```python
from build123d import *

# Parameters (mm, degrees)
SKETCH1_W           = 150
SKETCH1_H           = 150
BOSS_EXTRUDE1_DEPTH = 19
SKETCH2_R           = 28
CUT_EXTRUDE1_DEPTH  = 3
SKETCH3_R           = 2.5
CUT_EXTRUDE2_DEPTH  = 5
CIRPATTERN1_COUNT   = 4


with BuildPart() as part:
    # Sketch1 → Boss-Extrude1 (new body)
    with BuildSketch(Plane(origin=(0, 0, 0), x_dir=(1, 0, 0), z_dir=(0, 1, 0))):
        with Locations((75, 75)):
            Rectangle(SKETCH1_W, SKETCH1_H)
    extrude(amount=BOSS_EXTRUDE1_DEPTH)

    # Sketch2 → Cut-Extrude1 (cut)
    with BuildSketch(Plane(origin=(0, 19, 0), x_dir=(1, 0, 0), z_dir=(0, 1, 0))):
        with Locations((75, 75)):
            Circle(SKETCH2_R)
    extrude(amount=-CUT_EXTRUDE1_DEPTH, mode=Mode.SUBTRACT)

    # Sketch3 → Cut-Extrude2 (cut)
    with BuildSketch(Plane(origin=(0, 19, 0), x_dir=(1, 0, 0), z_dir=(0, 1, 0))):
        with Locations((100, 5)):
            Circle(SKETCH3_R)
        with Locations((50, 5)):
            Circle(SKETCH3_R)
    cut_extrude2 = extrude(amount=-CUT_EXTRUDE2_DEPTH, mode=Mode.SUBTRACT)

    # CirPattern1: Cut-Extrude2 ×4 about axis
    cirpattern1_axis = Axis((75, 0, -75), (0, 1, 0))
    for i in range(1, CIRPATTERN1_COUNT):
        add(cut_extrude2.rotate(cirpattern1_axis, i * 360 / CIRPATTERN1_COUNT), mode=Mode.SUBTRACT)


solid = part.part
```
Work out the finished part from the listing and answer in its coordinate system (mm). A direction names the side the tool comes from. Coordinates: 2 decimals unless noted, no trailing zeros. Write each loop counter-clockwise with the first axis right and the second up, starting at its lowest first coordinate (ties: lowest second). Pieces come first, ordered by that corner, then holes.
Q1. A cutting plane is placed at C-C, the plane z = -82.5. Give the vertices of the cut face in (x, y), then the cut area to 3 significant figures.
Q2. Find the intervals of material crossed by line 1 (Z direction, x = 145, y = 16.05); line 2 (X direction, y = 15.15, z = -5); line 3 (Z direction, x = 50, y = 15.65), in increasing order.
Q3. Each of these flat-tipped pins is pushed along its axis until it touches: pin 1 Ø6.5 at (x, z) = (145, -100) entering from -Y; pin 2 Ø1.5 at (x, z) = (100.5, -5.5) entering from +Y. Where does it stop, or does it pass through?
Q4. Which of the six approach directions +Z, -Z, +X, -X, +Y, -Y give full straight-line access (tool end or side, diameter ignored) to faces 5 (the face through (74, 9, 0)), 6 (the face through (75, 16, -75))?
Q5. A cutting plane is placed at B-B, the plane x = 75. Give the vertices of the cut face in (y, z).
Q6. A cutting plane is placed at A-A, the plane z = -145. Give the vertices of the cut face in (x, y).
Q7. Determine the mould class of faces 1 (the face through (102.385, 16.535, -5.751)), 2 (the face through (74, 0, -76)), 3 (the face through (150, 9, -74)), 4 (the face through (100.33, 16.54, -142.52)) for opening direction X: released by +X, released by -X, zero draft, split by the parting line, or undercut.
Q8. A cutting plane is placed at D-D, the plane x = 5. Give the vertices of the cut face in (y, z).
Findings below:
1. outline: (0, 0) - (150, 0) - (150, 19) - (101.98, 19) - (101.98, 16) - (48.02, 16) - (48.02, 19) - (0, 19) - close
1. area: 2,690 mm2
2. line 1: z = -150 to -102.5, -97.5 to -52.5, -47.5 to 0
2. line 2: x = 0 to 47.5, 52.5 to 97.5, 102.5 to 150
2. line 3: z = -150 to -147.5, -142.5 to -7.5, -2.5 to 0
3. pin 1: stops at y = 0
3. pin 2: stops at y = 14
4. face 5: +Z, +X, -X, +Y, -Y
4. face 6: +Y
5. outline: (0, -150) - (19, -150) - (19, -103) - (16, -103) - (16, -47) - (19, -47) - (19, 0) - (0, 0) - close
6. outline: (0, 0) - (150, 0) - (150, 19) - (102.5, 19) - (102.5, 14) - (97.5, 14) - (97.5, 19) - (52.5, 19) - (52.5, 14) - (47.5, 14) - (47.5, 19) - (0, 19) - close
7. face 1: undercut
7. face 2: zero draft
7. face 3: released by +X
7. face 4: undercut
8. outline: (0, -150) - (19, -150) - (19, -102.5) - (14, -102.5) - (14, -97.5) - (19, -97.5) - (19, -52.5) - (14, -52.5) - (14, -47.5) - (19, -47.5) - (19, 0) - (0, 0) - close
